```python
from build123d import *

# Parameters (mm, degrees)
SKETCH1_R               = 4
SKETCH1_R_2             = 2
BOSS_EXTRUDE1_DEPTH     = 20
CUT_EXTRUDE1_DEPTH      = 17
CUT_EXTRUDE1_DEPTH_BACK = 17
SKETCH3_R               = 4
CUT_EXTRUDE2_DEPTH      = 37
SKETCH4_R               = 1.395
CUT_EXTRUDE3_DEPTH      = 41
CUT_EXTRUDE4_DEPTH      = 4
FILLET1_R               = 3


with BuildPart() as part:
    # Sketch1 → Boss-Extrude1 (new body, symmetric)
    with BuildSketch(Plane.XY):
        with BuildLine():
            Line((-4.665710042, 7.69617761), (48.118899649, 39.69617761))
            ThreePointArc((48.118899649, 39.69617761), (53.543313423, 40.967963461), (58.676968473, 38.802948477))
            Line((58.676968473, 38.802948477), (97.36755541, 5.291182149))
            ThreePointArc((97.36755541, 5.291182149), (99.783371388, 0.131661326), (97.563318746, -5.115069869))
            Line((97.563318746, -5.115069869), (75.824988549, -25.423913737))
            Line((75.824988549, -25.423913737), (-1.882663558, -8.800885065))
            ThreePointArc((-1.882663558, -8.800885065), (-8.874602438, -1.497141134), (-4.665710042, 7.69617761))
        make_face()
        Circle(SKETCH1_R, mode=Mode.SUBTRACT)
        with Locations((84.784609691, 0)):
            Circle(SKETCH1_R, mode=Mode.SUBTRACT)
        with Locations((60.784609691, 0)):
            Circle(SKETCH1_R_2, mode=Mode.SUBTRACT)
        with Locations((52.784609691, -8)):
            Circle(SKETCH1_R_2, mode=Mode.SUBTRACT)
        with Locations((44.784609691, 0)):
            Circle(SKETCH1_R_2, mode=Mode.SUBTRACT)
        with Locations((52.784609691, 8)):
            Circle(SKETCH1_R_2, mode=Mode.SUBTRACT)
        with Locations((52.784609691, 32)):
            Circle(SKETCH1_R, mode=Mode.SUBTRACT)
    extrude(amount=BOSS_EXTRUDE1_DEPTH, both=True)

    # Sketch2 → Cut-Extrude1 (cut, two sides)
    with BuildSketch(Plane.XY) as cut_extrude1_sk:
        with BuildLine():
            Line((-4.665710042, 7.69617761), (39.891888688, 34.708656583))
            ThreePointArc((39.891888688, 34.708656583), (26.010438267, 4.38794834), (49.070722017, -19.700707237))
            Line((49.070722017, -19.700707237), (-1.882663558, -8.800885065))
            ThreePointArc((-1.882663558, -8.800885065), (-8.874602438, -1.497141134), (-4.665710042, 7.69617761))
        make_face()
    extrude(amount=CUT_EXTRUDE1_DEPTH, mode=Mode.SUBTRACT)
    extrude(cut_extrude1_sk.sketch, amount=-CUT_EXTRUDE1_DEPTH_BACK, mode=Mode.SUBTRACT)

    # Sketch3 → Cut-Extrude2 (cut)
    with BuildSketch(Plane(origin=(0, 0, -20), x_dir=(-1, 0, 0), z_dir=(0, 0, -1))):
        with Locations((-52.784609691, 8)):
            Circle(SKETCH3_R)
        with Locations((-60.784609691, 0)):
            Circle(SKETCH3_R)
        with Locations((-52.784609691, -8)):
            Circle(SKETCH3_R)
        with Locations((-44.784609691, 0)):
            Circle(SKETCH3_R)
    extrude(amount=-CUT_EXTRUDE2_DEPTH, mode=Mode.SUBTRACT)

    # Sketch4 → Cut-Extrude3 (cut, through all)
    with BuildSketch(Plane.XY.offset(20)):
        with Locations((33.650538517, 22.427469232)):
            Circle(SKETCH4_R)
    extrude(amount=-CUT_EXTRUDE3_DEPTH, mode=Mode.SUBTRACT)

    # Sketch5 → Cut-Extrude4 (cut)
    with BuildSketch(Plane(origin=(0, 0, -20), x_dir=(-1, 0, 0), z_dir=(0, 0, -1))):
        with BuildLine():
            Line((-97.36755541, 5.291182149), (-84.784609691, 16.189872762))
            ThreePointArc((-84.784609691, 16.189872762), (-68.601779215, -0.477470257), (-85.739134824, -16.161709743))
            Line((-85.739134824, -16.161709743), (-97.563318746, -5.115069869))
            ThreePointArc((-97.563318746, -5.115069869), (-99.783371388, 0.131661326), (-97.36755541, 5.291182149))
        make_face()
    extrude(amount=-CUT_EXTRUDE4_DEPTH, mode=Mode.SUBTRACT)

    # Fillet1
    fillet1_edges = [part.edges().sort_by_distance(p)[0] for p in [
        (84.784609691, 16.189872762, -18),
        (85.739134824, -16.161709743, -18),
    ]]
    fillet(fillet1_edges, radius=FILLET1_R)


solid = part.part
```
Read the model definition and answer for the solid it produces. Units are mm, in the model's axes. A direction names the side the tool comes from. Give positions to 0.01 mm unless a question says otherwise; leave off trailing zeros. Order: outer loops, then holes, each group sorted by start corner. A loop starts at its lowest first (then second) coordinate and runs counter-clockwise, first axis right, second up. Notation, with made-up numbers: (-32, -15) -> (18, -15) arc R27 cw to (18, 11) -> close; hole circle Ø11 at (20, 25). An arc over 180 degrees is marked (long way). One line per item, written item: value. Start each with the question number.
(1) The part is cut by section D-D (x = 27). Determine the outline of the cut face in (y, z).
(2) For a pull along Y with two mould halves and no side action, classify faces 6 (the cylindrical face through (54.692, -7.399, 18.479)), 7 (the flat face through (86.846, -15.127, 0.28)), 8 (the flat face through (41.2, 35.5, 0.1)) as released by +Y, released by -Y, zero draft, split by the parting line, or undercut.
(3) Straight lines are drawn through the part: L1, parallel to X at y = 0, z = 19.15; L2, parallel to X at y = 0.5, z = 12; L3, parallel to Z at x = 0.5, y = -4.5. For each, find the intervals that lie inside material, in ascending order.
(4) Flat-ended cylindrical pins translate along their axes: P1, Ø5, axis at x = 27.5, z = 7.5, coming from the -Y side; P2, Ø13, axis at x = 0, y = 0, coming from the -Z side; P3, Ø5, axis at x = 29.5, z = 1.5, coming from the -Y side; P4, Ø2, axis at y = 4, z = -5, coming from the -X side. Find the tip coordinate at first contact, or state that the pin passes through.
(5) The part is cut by section A-A (x = 0). Determine the outline of the cut face in (y, z).
(6) A tool of negligible diameter and unlimited length cuts with its end or side. For faces 1 (the cylindrical face through (25.93, 4.88, 0.24)), 2 (the cylindrical face through (54.935, 35.373, -0.28)), 3 (the cylindrical face through (81.062, 17.416, -17.972)), 4 (the cylindrical face through (-8.848, -1.645, -18.479)), 5 (the cylindrical face through (64.78, 0.18, -1.76)), from which of +Z, -Z, +X, -X, +Y, -Y can it reach the whole face along a straight path? Write none if from no direction.
(7) The part is cut by section B-B (z = -9). Determine the outline of the cut face in (x, y) (3 decimals).
(8) The part is cut by section C-C (y = 0). State how many separate pieces and enclosed holes the cut face has, and give its area (3 significant figures).
Taken from the geometry:
1. outline: (-14.98, -20) -> (26.89, -20) -> (26.89, -17) -> (18.34, -17) -> (18.34, 17) -> (26.89, 17) -> (26.89, 20) -> (-14.98, 20) -> (-14.98, 17) -> (0.31, 17) -> (0.31, -17) -> (-14.98, -17) -> close
2. face 6: undercut
2. face 7: released by -Y
2. face 8: released by +Y
3. L1: -9 to -4, 4 to 42.78, 46.78 to 58.78, 62.78 to 80.78, 88.78 to 99.78
3. L2: 26.94 to 40.82, 48.75 to 56.82, 64.75 to 80.82, 88.75 to 99.77
3. L3: -20 to -17, 17 to 20
4. P1: y = -6.23
4. P2: z = -20
4. P3: y = -9.09
4. P4: x = 25.91
5. outline: (-9.2, -20) -> (-4, -20) -> (-4, -17) -> (-9.2, -17) -> close; (-9.2, 17) -> (-4, 17) -> (-4, 20) -> (-9.2, 20) -> close; (4, -20) -> (10.52, -20) -> (10.52, -17) -> (4, -17) -> close; (4, 17) -> (10.52, 17) -> (10.52, 20) -> (4, 20) -> close
6. face 1: -X
6. face 2: +Z, -Z
6. face 3: -Z, +X
6. face 4: +Z, -Z, -X
6. face 5: -Z
7. outline: (39.892, 34.709) arc R29.683 ccw to (49.071, -19.701) -> (75.825, -25.424) -> (97.563, -5.115) arc R7 ccw to (97.368, 5.291) -> (58.677, 38.803) arc R9 ccw to (48.119, 39.696) -> close; hole circle Ø2.79 at (33.651, 22.427); hole circle Ø8 at (44.785, 0); hole circle Ø8 at (52.785, -8); hole circle Ø8 at (52.785, 8); hole circle Ø8 at (52.785, 32); hole circle Ø8 at (60.785, 0); hole circle Ø8 at (84.785, 0)
8. separate pieces: 6
8. enclosed holes: 0
8. area: 2,050 mm^2
